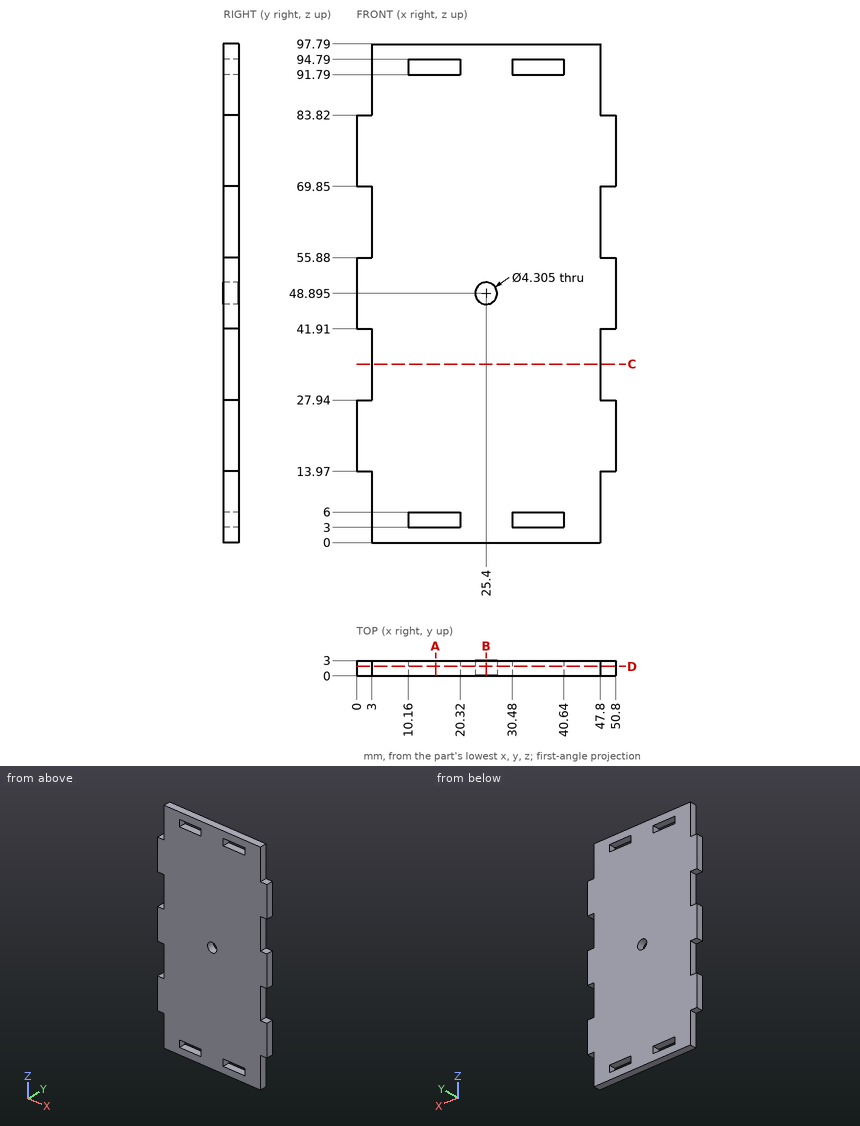
Answer from the drawing. Dimensions are ordinates in mm from the lowest x, y and z of the part. Round coordinates to 2 decimals unless told otherwise and drop trailing zeros. Loops run counter-clockwise (first coordinate to the right, second up) from the corner with the lowest first, then second, coordinate; pieces in that order, holes last.
(1) The part is cut by section C-C, the plane z = 35. Give the vertices of the cut face in (x, y).
Computed values:
outline: (3, 0) - (47.8, 0) - (47.8, 3) - (3, 3) - close
(2) Find the intervals of material crossed by L1, parallel to Z at x = 11, y = 2.5; L2, parallel to Z at x = 48, y = 2.1; L3, parallel to Z at x = 25.4, y = 1.8, in increasing order.
Computed values:
L1: z = 0 to 3, 6 to 91.79, 94.79 to 97.79
L2: z = 13.97 to 27.94, 41.91 to 55.88, 69.85 to 83.82
L3: z = 0 to 46.74, 51.05 to 97.79
(3) The part is cut by section B-B, the plane x = 25.4. Give the vertices of the cut face in (y, z).
Computed values:
outline: (0, 0) - (3, 0) - (3, 46.74) - (0, 46.74) - close; (0, 51.05) - (3, 51.05) - (3, 97.79) - (0, 97.79) - close
(4) The part is cut by section A-A, the plane x = 15.5. Give the vertices of the cut face in (y, z), and give its area (3 significant figures).
Computed values:
outline: (0, 0) - (3, 0) - (3, 3) - (0, 3) - close; (0, 6) - (3, 6) - (3, 91.79) - (0, 91.79) - close; (0, 94.79) - (3, 94.79) - (3, 97.79) - (0, 97.79) - close
area: 275 mm2
(5) Each of these flat-tipped pins is pushed along its axis until it touches: P1, Ø0.9, axis at y = 2, z = 6, coming from the -X side; P2, Ø12, axis at x = 25, z = 24.5, coming from the -Y side; P3, Ø1.5, axis at y = 2, z = 4, coming from the +X side; P4, Ø1.5, axis at x = 1, y = 1, coming from the +Z side. Where does it stop, or does it pass through?
Computed values:
P1: stops at x = 3
P2: stops at y = 0
P3: stops at x = 47.8
P4: stops at z = 83.82
(6) The part is cut by section D-D, the plane y = 1.9. Give the number of separate pieces and of enclosed holes in the cut face, and give its area (3 significant figures).
Computed values:
separate pieces: 1
enclosed holes: 5
area: 4,500 mm2
